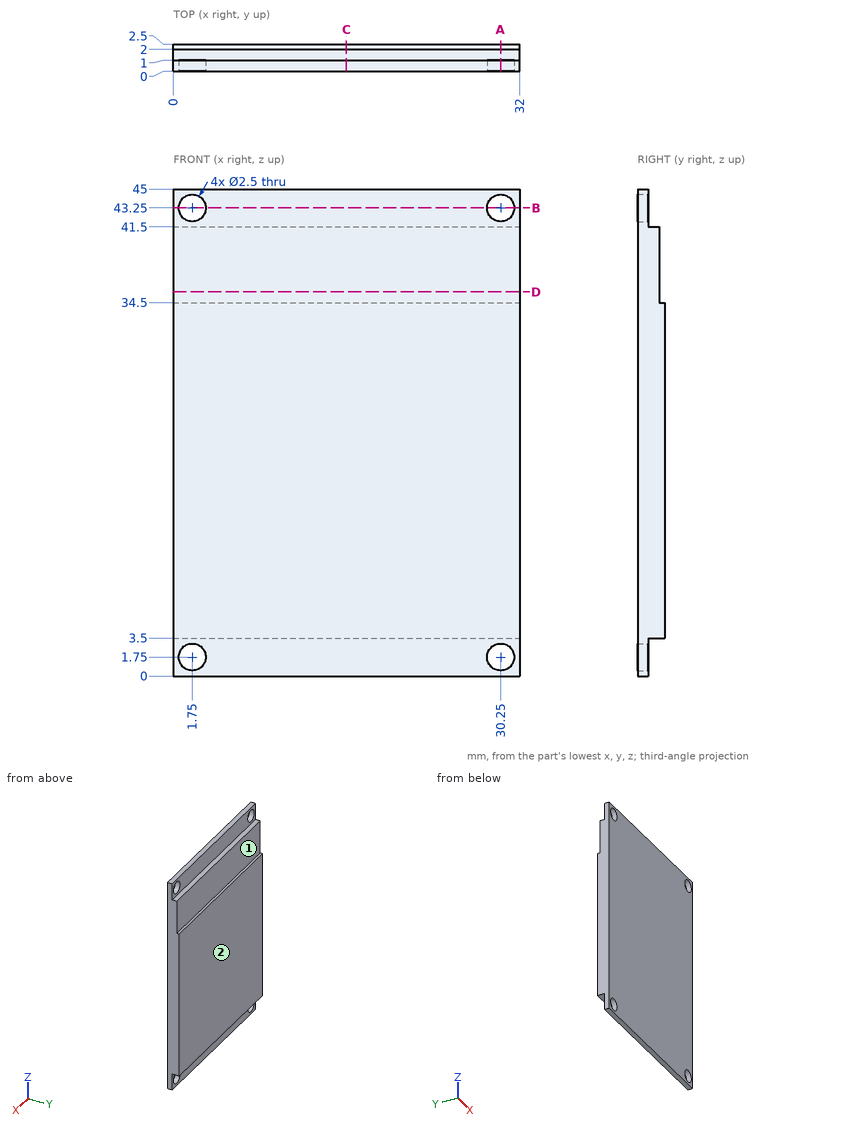
Drawing for the job (mm, zero at the part's lowest x, y, z). A direction names the side the tool comes from. Round coordinates to 2 decimals unless told otherwise and drop trailing zeros. Write each loop counter-clockwise with the first axis right and the second up, starting at its lowest first coordinate (ties: lowest second). Pieces come first, ordered by that corner, then holes. Notation, with made-up numbers: (-32, -7) - (-4, -7) arc R9 ccw to (-4, 0) - close; hole circle Ø7 at (-12.75, 3). An arc over 180 degrees is marked (long way). Write item = value, one per line. Start each with the question number.
Q1. Band-saw the part on B-B (z = 43.25). Give the cut face in (x, y), then the cut area to 3 significant figures.
Q2. Band-saw the part on A-A (x = 30.25). Give the cut face in (y, z), then the cut area to 3 significant figures.
Q3. Which spindle directions (+Z, -Z, +X, -X, +Y, -Y) get a long thin tool onto all of the face, cutting with end or side? Do the marked faces 1 and 2. Say none if no direction does.
Q4. Probe L1, parallel to X at y = 0.5, z = 43.25; L2, parallel to Z at x = 31, y = 0.75; L3, parallel to Z at x = 30.5, y = 0.5. List the from-to ranges inside material, lowest first. Write a range as from..to.
Q5. Drop flat-ended pins along their axis: pin 1 (0.8 mm diameter, centred on x = 23.5, y = 2, fed in from -Z); pin 2 (4 mm diameter, centred on x = 1.75, z = 43.25, fed in from +Y); pin 3 (4 mm diameter, centred on x = 30.25, z = 1.75, fed in from +Y); pin 4 (2 mm diameter, centred on x = 1.75, z = 1.75, fed in from +Y). Give the stop position or say it passes through.
Q6. Band-saw the part on D-D (z = 35.5). Give the cut face in (x, y), then the cut area to 3 significant figures.
Q7. Band-saw the part on C-C (x = 16). Give the cut face in (y, z), then the cut area to 3 significant figures.
Answers below:
q1.outline = (0, 0) - (0.5, 0) - (0.5, 1) - (0, 1) - close; (3, 0) - (29, 0) - (29, 1) - (3, 1) - close; (31.5, 0) - (32, 0) - (32, 1) - (31.5, 1) - close
q1.area = 27.0 mm2
q2.outline = (0, 0) - (1, 0) - (1, 0.5) - (0, 0.5) - close; (0, 3) - (1, 3) - (1, 3.5) - (2.5, 3.5) - (2.5, 34.5) - (2, 34.5) - (2, 41.5) - (1, 41.5) - (1, 42) - (0, 42) - close; (0, 44.5) - (1, 44.5) - (1, 45) - (0, 45) - close
q2.area = 93.5 mm2
q3.face_1 = +Z, +X, -X, +Y
q3.face_2 = +Z, -Z, +X, -X, +Y
q4.L1 = 0..0.5, 3..29, 31.5..32
q4.L2 = 0..0.75, 2.75..42.25, 44.25..45
q4.L3 = 0..0.53, 2.97..42.03, 44.47..45
q5.pin_1 = 3.5
q5.pin_2 = 2
q5.pin_3 = 2.5
q5.pin_4 = through
q6.outline = (0, 0) - (32, 0) - (32, 2) - (0, 2) - close
q6.area = 64.0 mm2
q7.outline = (0, 0) - (1, 0) - (1, 3.5) - (2.5, 3.5) - (2.5, 34.5) - (2, 34.5) - (2, 41.5) - (1, 41.5) - (1, 45) - (0, 45) - close
q7.area = 98.5 mm2
